Geometry: final body of the model. Coordinates: model frame, mm. Round coordinates to 2 decimals unless told otherwise and drop trailing zeros. Order: outer loops, then holes, each group sorted by start corner. A loop starts at its lowest first (then second) coordinate and runs counter-clockwise, first axis right, second up. Notation, with made-up numbers: M 42.25,-20 L 58.25,-20 A13 ccw 58.25,5 Z; hole C 30.25,-28.5 d4. An arc over 180 degrees is marked long. Put each result on its own line as item: value. Start each with the question number.
1) Section A-A, the plane x = -109. Return loops of the section in (y, z), then the cut area to 3 significant figures.
2) Section B-B, the plane x = -310. Return loops of the section in (y, z), then the cut area to 3 significant figures.
3) First-contact query: P1, Ø3.5, axis at x = -265, y = 63, coming from the -Z side; P2, Ø5.5, axis at x = -55, y = 63, coming from the -Z side; P3, Ø1, axis at y = -1.5, z = 3, coming from the +X side; P4, Ø2, axis at x = -84, z = 2, coming from the -Y side. Flat tips, straight axial feed; report the tip coordinate or a pass-through.
4) Material intervals for probe 1 along Y at (x, z) = (-195, 2.8); probe 2 along X at (y, z) = (21.5, 2.1); probe 3 along Y at (x, z) = (-145, 2.9), sorted ascending. Write a range as [from, to].
5) Section C-C, the plane z = 0.8. Count the separate pieces of the cut face and the enclosed holes in it, then the cut area to 3 significant figures.
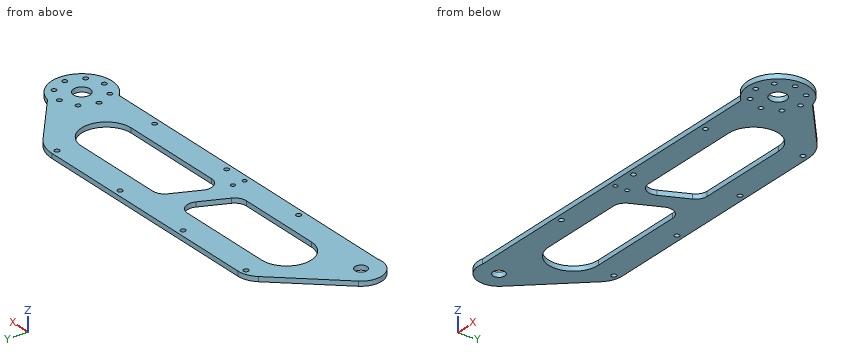
from build123d import *

# Parameters (mm, degrees)
SKETCH_2_R      = 2.1
SKETCH_2_R_2    = 1.75
SKETCH_2_R_3    = 5.03
SKETCH_2_R_4    = 2
SKETCH_2_R_5    = 7
EXTRUDE_1_DEPTH = 4


with BuildPart() as part:
    # 草图2 → 凸台-拉伸1 (new body)
    with BuildSketch(Plane.XY):
        with BuildLine():
            Line((-56.063767215, 68), (-262.305181408, 68))
            ThreePointArc((-262.305181408, 68), (-270.328158767, 66.320257484), (-277.003482509, 61.56318343))
            Line((-277.003482509, 61.56318343), (-322.861013463, 11.867785501))
            ThreePointArc((-322.861013463, 11.867785501), (-325.076248752, -8.885759595), (-305.846688069, -17))
            Line((-305.846688069, -17), (-19.006577809, -17))
            ThreePointArc((-19.006577809, -17), (22.016096561, -12.86629287), (5.482131266, 24.903739414))
            Line((5.482131266, 24.903739414), (-36.585436121, 60.816542635))
            ThreePointArc((-36.585436121, 60.816542635), (-45.683407853, 66.146902841), (-56.063767215, 68))
        make_face()
        with Locations((-225, -12)):
            Circle(SKETCH_2_R, mode=Mode.SUBTRACT)
        with Locations((-165, -12)):
            Circle(SKETCH_2_R_2, mode=Mode.SUBTRACT)
        with Locations((-310, 0)):
            Circle(SKETCH_2_R_3, mode=Mode.SUBTRACT)
        with Locations((-165, -2)):
            Circle(SKETCH_2_R_2, mode=Mode.SUBTRACT)
        with Locations((-145, -12)):
            Circle(SKETCH_2_R_4, mode=Mode.SUBTRACT)
        with Locations((-65, -12)):
            Circle(SKETCH_2_R_4, mode=Mode.SUBTRACT)
        with Locations((0, -19)):
            Circle(SKETCH_2_R_4, mode=Mode.SUBTRACT)
        with Locations((-13.435028843, -13.435028843)):
            Circle(SKETCH_2_R_4, mode=Mode.SUBTRACT)
        with Locations((13.435028843, -13.435028843)):
            Circle(SKETCH_2_R_4, mode=Mode.SUBTRACT)
        with Locations((-19, 0)):
            Circle(SKETCH_2_R_4, mode=Mode.SUBTRACT)
        Circle(SKETCH_2_R_5, mode=Mode.SUBTRACT)
        with Locations((19, 0)):
            Circle(SKETCH_2_R_4, mode=Mode.SUBTRACT)
        with Locations((-13.435028843, 13.435028843)):
            Circle(SKETCH_2_R_4, mode=Mode.SUBTRACT)
        with Locations((13.435028843, 13.435028843)):
            Circle(SKETCH_2_R_4, mode=Mode.SUBTRACT)
        with Locations((0, 19)):
            Circle(SKETCH_2_R_4, mode=Mode.SUBTRACT)
        with BuildLine():
            Line((-168.599525043, 31.773817383), (-178.858293522, 9.773817383))
            ThreePointArc((-178.858293522, 9.773817383), (-182.548375309, 5.566085542), (-187.921371393, 4))
            Line((-187.921371393, 4), (-260, 4))
            ThreePointArc((-260, 4), (-281, 25), (-260, 46))
            Line((-260, 46), (-177.662602913, 46))
            ThreePointArc((-177.662602913, 46), (-169.228688455, 41.372996083), (-168.599525043, 31.773817383))
        make_face(mode=Mode.SUBTRACT)
        with Locations((-265, 63)):
            Circle(SKETCH_2_R, mode=Mode.SUBTRACT)
        with Locations((-195, 63)):
            Circle(SKETCH_2_R, mode=Mode.SUBTRACT)
        with BuildLine():
            Line((-60, 4), (-149.303144229, 4))
            ThreePointArc((-149.303144229, 4), (-157.737058687, 8.627003917), (-158.366222099, 18.226182617))
            Line((-158.366222099, 18.226182617), (-148.10745362, 40.226182617))
            ThreePointArc((-148.10745362, 40.226182617), (-144.417371833, 44.433914458), (-139.044375749, 46))
            Line((-139.044375749, 46), (-60, 46))
            ThreePointArc((-60, 46), (-39, 25), (-60, 4))
        make_face(mode=Mode.SUBTRACT)
        with Locations((-125, 63)):
            Circle(SKETCH_2_R, mode=Mode.SUBTRACT)
        with Locations((-55, 63)):
            Circle(SKETCH_2_R, mode=Mode.SUBTRACT)
    extrude(amount=EXTRUDE_1_DEPTH)


solid = part.part
Result sheet:
1. outline: M -17,0 L 4,0 L 4,4 L -17,4 Z; M 46,0 L 68,0 L 68,4 L 46,4 Z
1. area: 172 mm2
2. outline: M -17.5,0 L -5.03,0 L -5.03,4 L -17.5,4 Z; M 5.03,0 L 25.81,0 L 25.81,4 L 5.03,4 Z
2. area: 133 mm2
3. P1: passes through
3. P2: stops at z = 0
3. P3: stops at x = 25.48
3. P4: stops at y = -17
4. probe 1: y = [-17, 4], [46, 60.9], [65.1, 68]
4. probe 2: x = [-313.97, -280.71], [-173.39, -156.84], [-39.29, 13.71]
4. probe 3: y = [-17, -14], [-10, 4], [44.03, 68]
5. separate pieces: 1
5. enclosed holes: 21
5. area: 16,900 mm2
